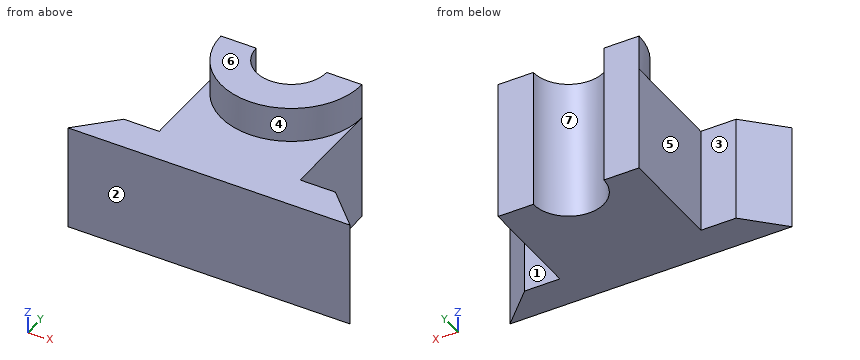
Autodesk Inventor part; units mm, degrees
ref_plane "YZ Plane" through (0, 0, 0) normal (1, 0, 0) x (0, 1, 0)
ref_plane "XZ Plane" through (0, 0, 0) normal (0, 1, 0) x (-1, 0, 0)
ref_plane "XY Plane" through (0, 0, 0) normal (0, 0, 1) x (1, 0, 0)
sketch "草圖1" plane through (0, 0, 0) normal (0, 0, 1) x (1, 0, 0)
  line L0 (-20, -5) -> (0, -5)
  line L1 (-20, -5) -> (-15, 0)
  line L2 (-15, 0) -> (-10, 0)
  line L3 (-10, 0) -> (-10, 15)
  line L4 (-10, 15) -> (0, 15)
  line L5 (0, -5) -> (0, 15)
  point P0 (0, 0)
  dimension "d0" = 20
  dimension "d1" = 5
  dimension "d2" = 5
  dimension "d3" = 20
  dimension "d4" = 10
extrude "擠出1" add sketch "草圖1" along normal mid plane 15
mirror "鏡射1" about plane through (0, -5, 0) normal (1, 0, 0) of "擠出1"
sketch "草圖2" plane through (0, 0, 7.5) normal (0, 0, 1) x (1, 0, 0)
  line L0 (-20, -5) -> (20, -5) construction
  line L1 (15, 0) -> (20, -5) construction
  line L2 (10, 0) -> (15, 0) construction
  line L3 (10, 15) -> (10, 0) construction
  line L4 (-10, 15) -> (10, 15) construction
  line L5 (-10, 15) -> (-10, 0) construction
  line L6 (-10, 0) -> (-15, 0) construction
  line L7 (-15, 0) -> (-20, -5) construction
  line L8 (-10, 15) -> (10, 15)
  arc A0 (-10, 15) -> (10, 15) centre (0, 15) ccw
  arc A1 (-5, 15) -> (5, 15) centre (0, 15) ccw
  point P0 (0, 0)
  dimension "d7" = 10
extrude "擠出2" add sketch "草圖2" along normal blind 5 contours L8 A1 A0
sketch "草圖3" plane through (0, 0, 7.5) normal (0, 0, 1) x (1, 0, 0)
  arc A0 (-5, 15) -> (5, 15) centre (0, 15) ccw
  line L0 (-5, 15) -> (5, 15)
  point P0 (0, 0)
extrude "擠出3" cut sketch "草圖3" against normal through all
properties part number "1"
Design review of the part built by this model. Coordinates are the model's own, in mm. Face numbers are marked on the shaded views. A direction names the side the tool comes from. Round coordinates to 2 decimals unless told otherwise and drop trailing zeros. Write each loop counter-clockwise with the first axis right and the second up, starting at its lowest first coordinate (ties: lowest second). Pieces come first, ordered by that corner, then holes. Notation, with made-up numbers: (-39.75, 28) -> (10.25, 28) arc R27 ccw to (10.25, 61) -> close; hole circle Ø6 at (63, 57.5). An arc over 180 degrees is marked (long way). One line per item, written item: value. Start each with the question number.
Q1. Add section B-B (x = 8). Give the boundary of the cut face in (y, z).
Q2. Add section C-C (y = 8.5). Give the boundary of the cut face in (x, z), then the cut area to 3 significant figures.
Q3. To check wall thickness, follow probe 1 along Z at (x, y) = (3.5, -3.75); probe 2 along X at (y, z) = (8.25, 0.75); probe 3 along X at (y, z) = (14, 11.25). State the ranges of each line that lie inside material, in increasing order.
Q4. The part is to be moulded in two halves that separate along X. For the marked faces 4, 5, 6 and 7, say which applies: pulls with the +X half, pulls with the -X half, needs draft (parallel to the pull), parting line crosses it, or undercut.
Q5. Add section D-D (y = 11.25). Give the boundary of the cut face in (x, z).
Q6. Insertion check: P1, Ø12, axis at y = 9, z = -0.5, coming from the -X side; P2, Ø4.5, axis at y = 8.5, z = 0.5, coming from the +X side; P3, Ø2.5, axis at x = -11.5, z = -3, coming from the +Y side. Each pin has a flat end and moves straight along its axis. Give the tip position at first contact, or say it passes through.
Q7. Add section A-A (z = -4.75). Give the boundary of the cut face in (x, y).
Q8. Tool access review of the marked faces 1, 2 and 3: name each direction out of +Z, -Z, +X, -X, +Y, -Y from which nothing blocks a thin tool from reaching the whole face with its end or side.
Response:
1. outline: (-5, -7.5) -> (15, -7.5) -> (15, 12.5) -> (9, 12.5) -> (9, 7.5) -> (-5, 7.5) -> close
2. outline: (-10, -7.5) -> (10, -7.5) -> (10, 7.5) -> (7.6, 7.5) -> (7.6, 12.5) -> (-7.6, 12.5) -> (-7.6, 7.5) -> (-10, 7.5) -> close
2. area: 376 mm^2
3. probe 1: z = -7.5 to 7.5
3. probe 2: x = -10 to 10
3. probe 3: x = -9.95 to -4.9, 4.9 to 9.95
4. face 4: parting line crosses it
4. face 5: pulls with the -X half
4. face 6: needs draft
4. face 7: undercut
5. outline: (-10, -7.5) -> (-3.31, -7.5) -> (-3.31, 12.5) -> (-9.27, 12.5) -> (-9.27, 7.5) -> (-10, 7.5) -> close; (3.31, -7.5) -> (10, -7.5) -> (10, 7.5) -> (9.27, 7.5) -> (9.27, 12.5) -> (3.31, 12.5) -> close
6. P1: stops at x = -10
6. P2: stops at x = 10
6. P3: stops at y = 0
7. outline: (-20, -5) -> (20, -5) -> (15, 0) -> (10, 0) -> (10, 15) -> (5, 15) arc R5 cw to (-5, 15) -> (-10, 15) -> (-10, 0) -> (-15, 0) -> close
8. face 1: +Z, -Z, +X, +Y
8. face 2: +Z, -Z, +X, -X, -Y
8. face 3: +Z, -Z, -X, +Y
